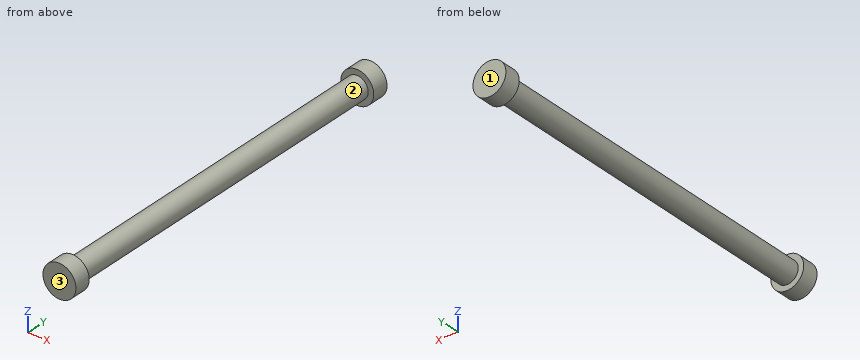
from build123d import *

# Parameters (mm, degrees)
F0_R     = 6.35
F1_DEPTH = 101.6
F2_R     = 9.525
F3_DEPTH = 9.525
F4_R     = 9.525
F5_DEPTH = 9.525


with BuildPart() as f1:
    # F0 (on Front) → F1 (new body, symmetric)
    with BuildSketch(Plane.XZ):
        Circle(F0_R)
    extrude(amount=F1_DEPTH, both=True)

    # F2 (on face) → F3 (join)
    with BuildSketch(Plane.XZ.offset(101.6)):
        Circle(F2_R)
    extrude(amount=F3_DEPTH)

    # F4 (on face) → F5 (join)
    with BuildSketch(Plane(origin=(0, 101.6, 0), x_dir=(-1, 0, 0), z_dir=(0, 1, 0))):
        Circle(F4_R)
    extrude(amount=F5_DEPTH)


solid = f1.part
Design review of the part built by this model. Coordinates are the model's own, in mm. Face numbers are marked on the shaded views. Give positions to 0.01 mm unless a question says otherwise; leave off trailing zeros. Loops run counter-clockwise (first coordinate to the right, second up) from the corner with the lowest first, then second, coordinate; pieces in that order, holes last. Notation, with made-up numbers: M 37.25,59 L 41.25,59 A33 cw 41.25,94 Z; hole C 67.25,-35 d11. An arc over 180 degrees is marked long. One line per question, with ' | ' between items. Start each with the question number.
1. Add section B-B (x = 0). Write out the cut boundary in (y, z) (3 decimals), plus the area to 3 significant figures.
2. Add section A-A (z = 0). Write out the cut boundary in (x, y) (3 decimals).
3. To check wall thickness, follow L1, parallel to Y at x = -3.5, z = -6.5 (3 decimals); L2, parallel to X at y = -84.5, z = 0.25; L3, parallel to Z at x = 0.5, y = 53.5. State the ranges of each line that lie inside material, in increasing order.
4. Insertion check: P1, Ø10, axis at x = 7.5, y = 14, coming from the -Z side; P2, Ø1.5, axis at y = -61.5, z = -4, coming from the -X side; P3, Ø1, axis at y = -61, z = -2.5, coming from the +X side. Each pin has a flat end and moves straight along its axis. Give the tip position at first contact, or say it passes through.
5. The part is to be moulded in two halves that separate along Y. For the marked faces 1, 2 and 3, say which applies: released by +Y, released by -Y, zero draft, split by the parting line, or undercut.
6. Add section C-C (y = 42.5). Write out the cut boundary in (x, z).
Worked out:
1) outline: M -111.125,-9.525 L -101.6,-9.525 L -101.6,-6.35 L 101.6,-6.35 L 101.6,-9.525 L 111.125,-9.525 L 111.125,9.525 L 101.6,9.525 L 101.6,6.35 L -101.6,6.35 L -101.6,9.525 L -111.125,9.525 Z | area: 2,940 mm²
2) outline: M -9.525,-111.125 L 9.525,-111.125 L 9.525,-101.6 L 6.35,-101.6 L 6.35,101.6 L 9.525,101.6 L 9.525,111.125 L -9.525,111.125 L -9.525,101.6 L -6.35,101.6 L -6.35,-101.6 L -9.525,-101.6 Z
3) L1: y = -111.125 to -101.6, 101.6 to 111.125 | L2: x = -6.35 to 6.35 | L3: z = -6.33 to 6.33
4) P1: stops at z = -5.84 | P2: stops at x = -5.46 | P3: stops at x = 6.03
5) face 1: released by +Y | face 2: undercut | face 3: released by -Y
6) outline: C 0,0 d12.7
